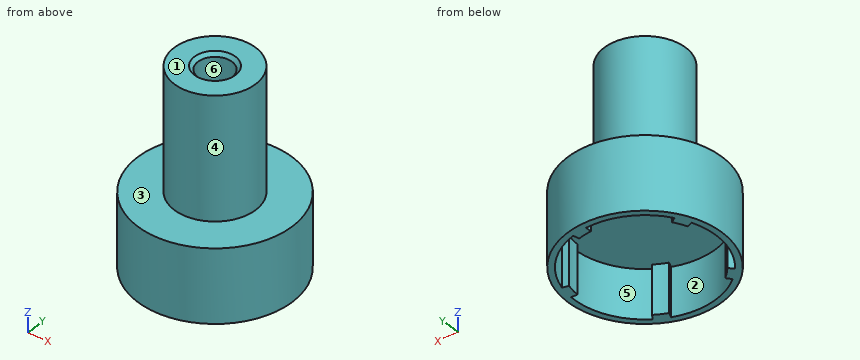
from build123d import *

# Parameters (mm, degrees)
SKETCH1_R                   = 9.5
SKETCH1_R_2                 = 8
BOSS_EXTRUDE1_DEPTH         = 6
SKETCH2_R                   = 9.5
BOSS_EXTRUDE2_DEPTH         = 3
SKETCH3_R                   = 5
BOSS_EXTRUDE3_DEPTH         = 15
CUT_EXTRUDE1_DEPTH          = 6
CIRPATTERN1_COUNT           = 5
M5_TAPPED_HOLE1_D           = 4.2
M5_TAPPED_HOLE1_DEPTH       = 15
M5_TAPPED_HOLE1_CSINK_D     = 5.05
M5_TAPPED_HOLE1_CSINK_ANGLE = 90
M5_TAPPED_HOLE1_TIP         = 1.2618073


with BuildPart() as part:
    # Sketch1 → Boss-Extrude1 (new body)
    with BuildSketch(Plane.XY):
        Circle(SKETCH1_R)
        Circle(SKETCH1_R_2, mode=Mode.SUBTRACT)
    extrude(amount=BOSS_EXTRUDE1_DEPTH)

    # Sketch2 → Boss-Extrude2 (add)
    with BuildSketch(Plane.XY.offset(6)):
        Circle(SKETCH2_R)
    extrude(amount=BOSS_EXTRUDE2_DEPTH)

    # Sketch3 → Boss-Extrude3 (add)
    with BuildSketch(Plane.XY.offset(9)):
        Circle(SKETCH3_R)
    extrude(amount=BOSS_EXTRUDE3_DEPTH)

    # Sketch4 → Cut-Extrude1 (cut)
    with BuildSketch(Plane(origin=(0, 0, 0), x_dir=(-1, 0, 0), z_dir=(0, 0, -1))):
        with BuildLine():
            Line((-7.72740661, 2.070552361), (-8.45185098, 2.264666645))
            ThreePointArc((-8.45185098, 2.264666645), (-6.187184335, 6.187184335), (-2.264666645, 8.45185098))
            Line((-2.264666645, 8.45185098), (-2.070552361, 7.72740661))
            ThreePointArc((-2.070552361, 7.72740661), (-5.656854249, 5.656854249), (-7.72740661, 2.070552361))
        make_face()
    cut_extrude1 = extrude(amount=-CUT_EXTRUDE1_DEPTH, mode=Mode.SUBTRACT)

    # CirPattern1: Cut-Extrude1 ×5 about axis
    cirpattern1_axis = Axis((0, 0, 0), (0, 0, 1))
    for i in range(1, CIRPATTERN1_COUNT):
        add(cut_extrude1.rotate(cirpattern1_axis, i * 360 / CIRPATTERN1_COUNT), mode=Mode.SUBTRACT)

    # M5 Tapped Hole1
    with Locations(Plane.XY.offset(24)):
        with Locations((0, 0)):
            CounterSinkHole(M5_TAPPED_HOLE1_D / 2, M5_TAPPED_HOLE1_CSINK_D / 2, depth=M5_TAPPED_HOLE1_DEPTH, counter_sink_angle=M5_TAPPED_HOLE1_CSINK_ANGLE)
            with Locations((0, 0, -(M5_TAPPED_HOLE1_DEPTH + M5_TAPPED_HOLE1_TIP / 2))):  # 118° drill point
                Cone(0, M5_TAPPED_HOLE1_D / 2, M5_TAPPED_HOLE1_TIP, mode=Mode.SUBTRACT)


solid = part.part
Geometry check sheet. Reference: the model listing, model coordinates, mm. Face numbers are marked on the shaded views. A direction names the side the tool comes from. Give positions to 0.01 mm unless a question says otherwise; leave off trailing zeros. Loops run counter-clockwise (first coordinate to the right, second up) from the corner with the lowest first, then second, coordinate; pieces in that order, holes last. Notation, with made-up numbers: M 50,43 L 82,43 A23 cw 82,62 Z; hole C -4,4 d5. An arc over 180 degrees is marked long. Write each question's results on one line, items separated by ' | '.
1) Gauge pin test, flat ends, axial feed: pin 1 (10 mm diameter, centred on y = -5, z = 12.5, fed in from +X); pin 2 (2 mm diameter, centred on y = -1.5, z = 16.5, fed in from +X); pin 3 (1 mm diameter, centred on x = -1.5, y = 4.5, fed in from -Z). Record the tip position at first contact, or that the pin passes through.
Answers follow:
pin 1: x = 9.39 | pin 2: x = 4.97 | pin 3: z = 6
2) Release check for a two-part mould opening along X. For the marked faces 3, 4, 5 and 6 record: +X half, -X half, draft (parallel to the pull), parting line (faces both ways), or undercut.
Answers follow:
face 3: draft | face 4: parting line | face 5: undercut | face 6: undercut
3) Section check D-D, the plane y = -4. Record the boundary of the cut face in (x, z), plus the area to 3 significant figures.
Answers follow:
outline: M -8.62,0 L -7.78,0 L -7.78,6 L 7.78,6 L 7.78,0 L 8.62,0 L 8.62,9 L 3,9 L 3,24 L -3,24 L -3,9 L -8.62,9 Z | area: 152 mm2
4) Tool access check on the marked faces 1 and 2. Record the directions out of +Z, -Z, +X, -X, +Y, -Y that give a thin tool (end or side, any length) a straight path to the whole face; none if there is none.
Answers follow:
face 1: +Z, +X, -X, +Y, -Y | face 2: -Z
5) Thickness scan on line 1 (Z direction, x = 3, y = -7); line 2 (X direction, y = -7.25, z = 3.5); line 3 (Y direction, x = 0, z = 16.5). Record the ranges inside material, lowest first.
Answers follow:
line 1: 6 to 9 | line 2: -6.14 to -4.9, 3.38 to 4.71, 4.9 to 6.14 | line 3: -5 to -2.1, 2.1 to 5
6) Section check B-B, the plane x = 6.25. Record the boundary of the cut face in (y, z), plus the area to 3 significant figures.
Answers follow:
outline: M -7.15,0 L -6.12,0 L -6.12,6 L 6.12,6 L 6.12,0 L 7.15,0 L 7.15,9 L -7.15,9 Z | area: 55.3 mm2
7) Section check A-A, the plane z = 4.25. Record the boundary of the cut face in (x, y).
Answers follow:
outline: C 0,0 d19; hole M -8.17,3.14 A8.75 ccw -6.8,-5.51 L -6.22,-5.03 A8 ccw -5.03,-6.22 L -5.51,-6.8 A8.75 ccw 3.14,-8.17 L 2.87,-7.47 A8 ccw 4.36,-6.71 L 4.77,-7.34 A8.75 ccw 8.74,0.46 L 7.99,0.42 A8 ccw 7.73,2.07 L 8.45,2.26 A8.75 ccw 2.26,8.45 L 2.07,7.73 A8 ccw 0.42,7.99 L 0.46,8.74 A8.75 ccw -7.34,4.77 L -6.71,4.36 A8 ccw -7.47,2.87 Z
8) Section check C-C, the plane z = 6.75. Record the boundary of the cut face in (x, y).
Answers follow:
outline: C 0,0 d19
